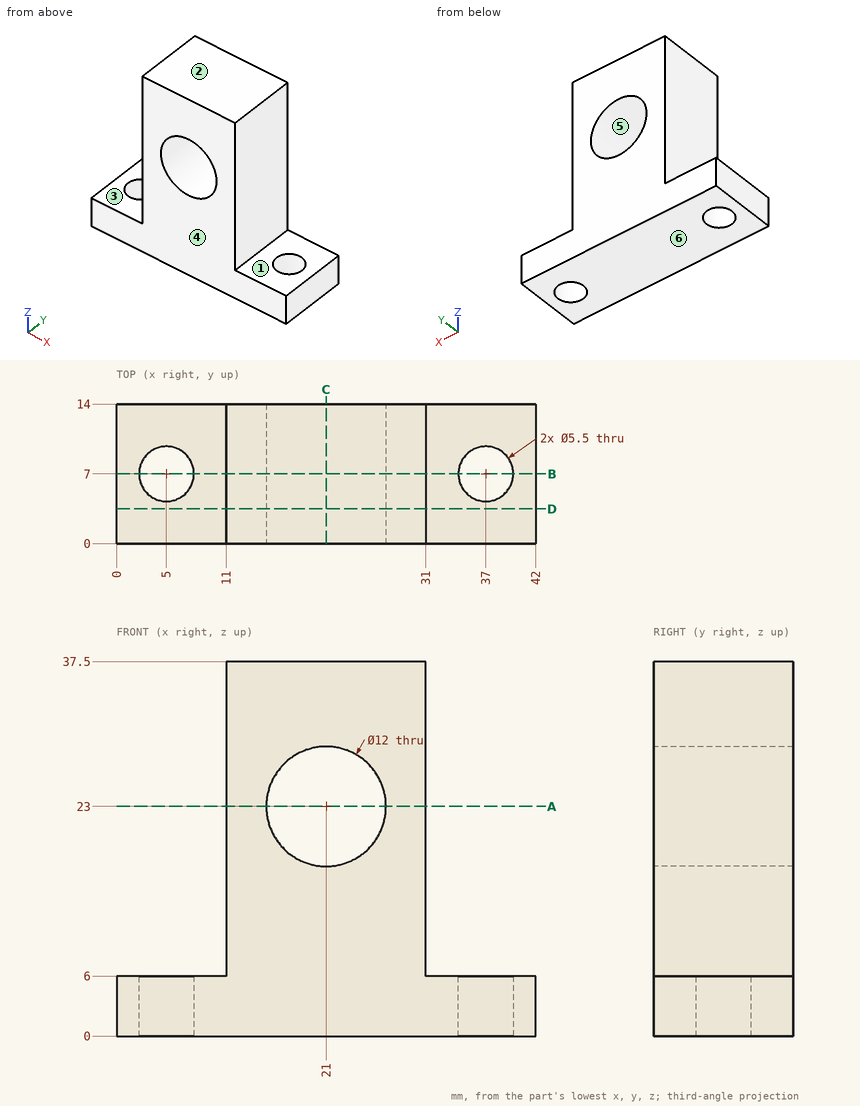
Geometry: see drawing. Coordinates: mm, zero at the bounding-box minimum. A direction names the side the tool comes from. Round coordinates to 2 decimals unless told otherwise and drop trailing zeros. Write each loop counter-clockwise with the first axis right and the second up, starting at its lowest first coordinate (ties: lowest second). Pieces come first, ordered by that corner, then holes.
Item 1: Set-up query: the marked faces 1, 2 and 3. Return all of +Z, -Z, +X, -X, +Y, -Y with unobstructed straight access to the full face (end or side cutting, diameter ignored); none if empty.
Item 2: Pin query (flat end, axial travel): P1, Ø7, axis at y = 5.5, z = 23, coming from the -X side; P2, Ø1, axis at y = 3, z = 7, coming from the +X side; P3, Ø4, axis at x = 35, y = 5, coming from the +Z side; P4, Ø3.5, axis at x = 37, y = 7, coming from the +Z side. Return the tip coordinate at first contact, or that it passes through.
Item 3: Section query B-B (y = 7). Return loops of the section in (x, z).
Item 4: Section query D-D (y = 3.5). Return loops of the section in (x, z), plus the area to 3 significant figures.
Item 5: Section query C-C (x = 21). Return loops of the section in (y, z).
Item 6: Material intervals for L1, parallel to Z at x = 21, y = 5.5; L2, parallel to Y at x = 37, z = 2; L3, parallel to X at y = 2.75, z = 9.5, sorted ascending.
Item 7: Section query A-A (z = 23). Return loops of the section in (x, y).
Item 8: Mould query, pull axis Z, two halves, no side actions, for the marked faces 4, 5 and 6. Classes: +Z half, -Z half, draft (parallel to the pull), parting line (faces both ways), or undercut.
Completed:
1. face 1: +Z, +X, +Y, -Y
1. face 2: +Z, +X, -X, +Y, -Y
1. face 3: +Z, -X, +Y, -Y
2. P1: stops at x = 11
2. P2: stops at x = 31
2. P3: stops at z = 6
2. P4: passes through
3. outline: (0, 0) - (2.25, 0) - (2.25, 6) - (0, 6) - close; (7.75, 0) - (34.25, 0) - (34.25, 6) - (31, 6) - (31, 37.5) - (11, 37.5) - (11, 6) - (7.75, 6) - close; (39.75, 0) - (42, 0) - (42, 6) - (39.75, 6) - close; hole circle Ø12 at (21, 23)
4. outline: (0, 0) - (42, 0) - (42, 6) - (31, 6) - (31, 37.5) - (11, 37.5) - (11, 6) - (0, 6) - close; hole circle Ø12 at (21, 23)
4. area: 769 mm2
5. outline: (0, 0) - (14, 0) - (14, 17) - (0, 17) - close; (0, 29) - (14, 29) - (14, 37.5) - (0, 37.5) - close
6. L1: z = 0 to 17, 29 to 37.5
6. L2: y = 0 to 4.25, 9.75 to 14
6. L3: x = 11 to 31
7. outline: (11, 0) - (15, 0) - (15, 14) - (11, 14) - close; (27, 0) - (31, 0) - (31, 14) - (27, 14) - close
8. face 4: draft
8. face 5: undercut
8. face 6: -Z half
